Read the model definition and answer for the solid it produces. Units are mm, in the model's axes. A direction names the side the tool comes from. Give positions to 0.01 mm unless a question says otherwise; leave off trailing zeros. Loops run counter-clockwise (first coordinate to the right, second up) from the corner with the lowest first, then second, coordinate; pieces in that order, holes last.
(1) Each of these flat-tipped pins is pushed along its axis until it touches: P1, Ø1.3, axis at x = 6, z = 10, coming from the -Y side; P2, Ø8, axis at x = 6.5, y = 33.5, coming from the +Z side. Where does it stop, or does it pass through?
(2) Which of the six approach directions +Z, -Z, +X, -X, +Y, -Y give full straight-line access (tool end or side, diameter ignored) to faces 5 (the face through (5, 23.661, 3)), 6 (the face through (-2, 40, 5)), 7 (the face through (28.2, 54, 8)), 8 (the face through (28.4, 24, 9))?
(3) Find section D-D, the plane z = 1.25. Write down the section's boundary in (x, y).
(4) Find section B-B, the plane y = 54. Write down the section's boundary in (x, z), then the cut area to 3 significant figures.
(5) Find section C-C, the plane x = -3. Write down the section's boundary in (y, z).
(6) Determine the mould class of faces 1 (the face through (-4, 54, 9.346)), 2 (the face through (5, 23.661, 10)), 3 (the face through (-4, 54, 6.846)), 4 (the face through (-2, 39, 0)) for opening direction Z: pulls with the +Z half, pulls with the -Z half, needs draft (parallel to the pull), parting line crosses it, or undercut.
(7) Find section A-A, the plane x = 4. Write down the section's boundary in (y, z).
(8) Straight lines are drawn through the part: probe 1 along X at (y, z) = (21, 10.75); probe 2 along Y at (x, z) = (10, 7); probe 3 along Y at (x, z) = (-21.5, 9.5). For each, find the intervals that lie inside material, in ascending order.
```python
from build123d import *

# Parameters (mm, degrees)
F0_R          = 1.6
F0_W          = 70
F0_H          = 9
F0_H_2        = 26.5
F1_DEPTH      = 11
F2_START      = 5
F2_DEPTH      = 6
F3_DEPTH      = 11
F4_W          = 2.5
F4_H          = 2.5
F4_W_2        = 5
F5_DEPTH      = 59.9
F5_DEPTH_BACK = 28.2
F7_START      = 28.4
F6_R          = 1.25
F7_DEPTH      = 20.7


with BuildPart() as f1:
    # F0 (on Top) → F1 (new body)
    with BuildSketch(Plane.XY):
        Polygon((33.6174106598, 26.1609371045), (-36.3825893402, 26.1609371045), (-36.3825893402, 16.6609371045), (0.1174106598, 16.6609371045), (0.1174106598, 23.6609371045), (9.1174106598, 23.6609371045), (9.1174106598, 16.6609371045), (33.6174106598, 16.6609371045), align=None)
        with Locations((-26.8825893402, 20.6609371045)):
            Circle(F0_R, mode=Mode.SUBTRACT)
        with Locations((24.1174106598, 20.6609371045)):
            Circle(F0_R, mode=Mode.SUBTRACT)
        with Locations((-1.3825893402, 57.1609371045)):
            Rectangle(F0_W, F0_H)
        with Locations((-1.3825893402, 39.4109371045)):
            Rectangle(F0_W, F0_H_2)
    extrude(amount=F1_DEPTH)

    # F0 (on Top) → F2 (cut)
    with BuildSketch(Plane.XY.offset(F2_START)):
        with Locations((-1.3825893402, 39.4109371045)):
            Rectangle(F0_W, F0_H_2)
    extrude(amount=F2_DEPTH, mode=Mode.SUBTRACT)

    # F0 (on Top) → F3 (join)
    with BuildSketch(Plane.XY):
        with Locations((-1.3825893402, 57.1609371045)):
            Rectangle(F0_W, F0_H)
    extrude(amount=F3_DEPTH)

    # F4 (on Right) → F5 (cut, two sides)
    with BuildSketch(Plane.YZ) as f5_sk:
        with Locations((53.8876638908, 8.095925469)):
            Rectangle(F4_W, F4_H)
        with Locations((25.6764949858, 8.095925469)):
            Rectangle(F4_W_2, F4_H)
    extrude(amount=-F5_DEPTH, mode=Mode.SUBTRACT)
    extrude(f5_sk.sketch, amount=F5_DEPTH_BACK, mode=Mode.SUBTRACT)

    # F6 (on Right) → F7 (cut)
    with BuildSketch(Plane.YZ.offset(F7_START)):
        with Locations((23.6609371045, 8.6017483845)):
            Circle(F6_R)
    extrude(amount=F7_DEPTH, mode=Mode.SUBTRACT)


solid = f1.part
```
Entries:
1. P1: stops at y = 23.66
1. P2: stops at z = 5
2. face 5: +Z, -Z, -Y
2. face 6: +Z, +X, -X
2. face 7: -X
2. face 8: +X
3. outline: (-36.38, 16.66) - (0.12, 16.66) - (0.12, 23.66) - (9.12, 23.66) - (9.12, 16.66) - (33.62, 16.66) - (33.62, 61.66) - (-36.38, 61.66) - close; hole circle Ø3.2 at (-26.88, 20.66); hole circle Ø3.2 at (24.12, 20.66)
4. outline: (-36.38, 0) - (33.62, 0) - (33.62, 11) - (-36.38, 11) - (-36.38, 9.35) - (28.2, 9.35) - (28.2, 6.85) - (-36.38, 6.85) - close
4. area: 609 mm2
5. outline: (16.66, 0) - (61.66, 0) - (61.66, 11) - (52.66, 11) - (52.66, 9.35) - (55.14, 9.35) - (55.14, 6.85) - (52.66, 6.85) - (52.66, 5) - (26.16, 5) - (26.16, 6.85) - (23.18, 6.85) - (23.18, 9.35) - (26.16, 9.35) - (26.16, 11) - (16.66, 11) - close
6. face 1: undercut
6. face 2: needs draft
6. face 3: undercut
6. face 4: pulls with the -Z half
7. outline: (23.66, 0) - (61.66, 0) - (61.66, 11) - (52.66, 11) - (52.66, 9.35) - (55.14, 9.35) - (55.14, 6.85) - (52.66, 6.85) - (52.66, 5) - (26.16, 5) - (26.16, 6.85) - (23.66, 6.85) - close; (23.66, 9.35) - (26.16, 9.35) - (26.16, 11) - (23.66, 11) - close
8. probe 1: x = -36.38 to -28.45, -25.32 to 0.12, 9.12 to 22.55, 25.68 to 33.62
8. probe 2: y = 16.66 to 23.18, 55.14 to 61.66
8. probe 3: y = 16.66 to 26.16, 52.66 to 61.66
